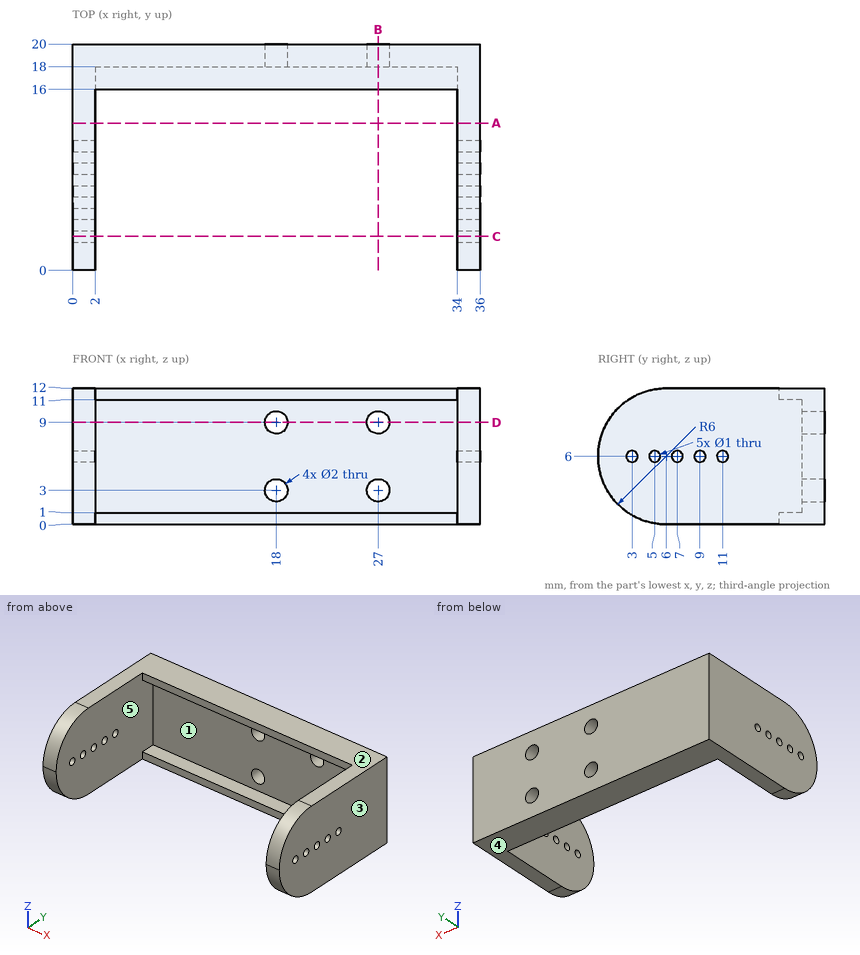
Geometry: see drawing. Coordinates: mm, zero at the bounding-box minimum. A direction names the side the tool comes from. Give positions to 0.01 mm unless a question says otherwise; leave off trailing zeros. Write each loop counter-clockwise with the first axis right and the second up, starting at its lowest first coordinate (ties: lowest second). Pieces come first, ordered by that corner, then holes. Notation, with made-up numbers: M 54,71 L 58,71 A17 cw 58,76 Z; hole C -14,-13.5 d5. An arc over 180 degrees is marked long. Return JSON: item names as keys, results as strings. Group by question number.
1) Set-up query: the marked faces 1 and 2. Return all of +Z, -Z, +X, -X, +Y, -Y with unobstructed straight access to the full face (end or side cutting, diameter ignored); none if empty.
2) Cut plane B-B, the plane x = 27. Output: boundary loops of the cut face in (y, z), then the cut area to 3 significant figures.
3) Ray query, L1, parallel to X at y = 18.7, z = 3; L2, parallel to Z at x = 23, y = 16.5; L3, parallel to X at y = 12, z = 4.5. Return the intervals inside material, ascending.
4) Cut plane A-A, the plane y = 13. Output: boundary loops of the cut face in (x, z), then the cut area to 3 significant figures.
5) First-contact query: pin 1 Ø0.8 at (x, z) = (15.5, 11.5) entering from -Y; pin 2 Ø8 at (x, y) = (25, 15) entering from +Z; pin 3 Ø2.5 at (x, z) = (27, 3) entering from -Y; pin 4 Ø1.6 at (x, z) = (27, 9) entering from +Y. Flat tips, straight axial feed; report the tip coordinate or a pass-through.
6) Cut plane C-C, the plane y = 3. Output: boundary loops of the cut face in (x, z), then the cut area to 3 significant figures.
7) Draft query along X for the marked faces 3, 4 and 5. Return one class per face: released by +X, released by -X, zero draft, split by the parting line, or undercut.
8) Cut plane D-D, the plane z = 9. Output: boundary loops of the cut face in (x, y).
Data:
{
 "1": {"face 1": "-Y", "face 2": "+Z, +X, -X, +Y, -Y"},
 "2": {"outline": "M 16,0 L 20,0 L 20,2 L 18,2 L 18,1 L 16,1 Z; M 16,11 L 18,11 L 18,10 L 20,10 L 20,12 L 16,12 Z; M 18,4 L 20,4 L 20,8 L 18,8 Z", "area": "20.0 mm²"},
 "3": {"L1": "x = 0 to 17, 19 to 26, 28 to 36", "L2": "z = 0 to 1, 11 to 12", "L3": "x = 0 to 2, 34 to 36"},
 "4": {"outline": "M 0,0 L 2,0 L 2,12 L 0,12 Z; M 34,0 L 36,0 L 36,12 L 34,12 Z", "area": "48.0 mm²"},
 "5": {"pin 1": "stops at y = 16", "pin 2": "stops at z = 12", "pin 3": "stops at y = 18", "pin 4": "passes through"},
 "6": {"outline": "M 0,0.8 L 2,0.8 L 2,5.5 L 0,5.5 Z; M 0,6.5 L 2,6.5 L 2,11.2 L 0,11.2 Z; M 34,0.8 L 36,0.8 L 36,5.5 L 34,5.5 Z; M 34,6.5 L 36,6.5 L 36,11.2 L 34,11.2 Z", "area": "37.6 mm²"},
 "7": {"face 3": "released by +X", "face 4": "zero draft", "face 5": "undercut"},
 "8": {"outline": "M 0,0.8 L 2,0.8 L 2,18 L 17,18 L 17,20 L 0,20 Z; M 19,18 L 26,18 L 26,20 L 19,20 Z; M 28,18 L 34,18 L 34,0.8 L 36,0.8 L 36,20 L 28,20 Z"}
}
